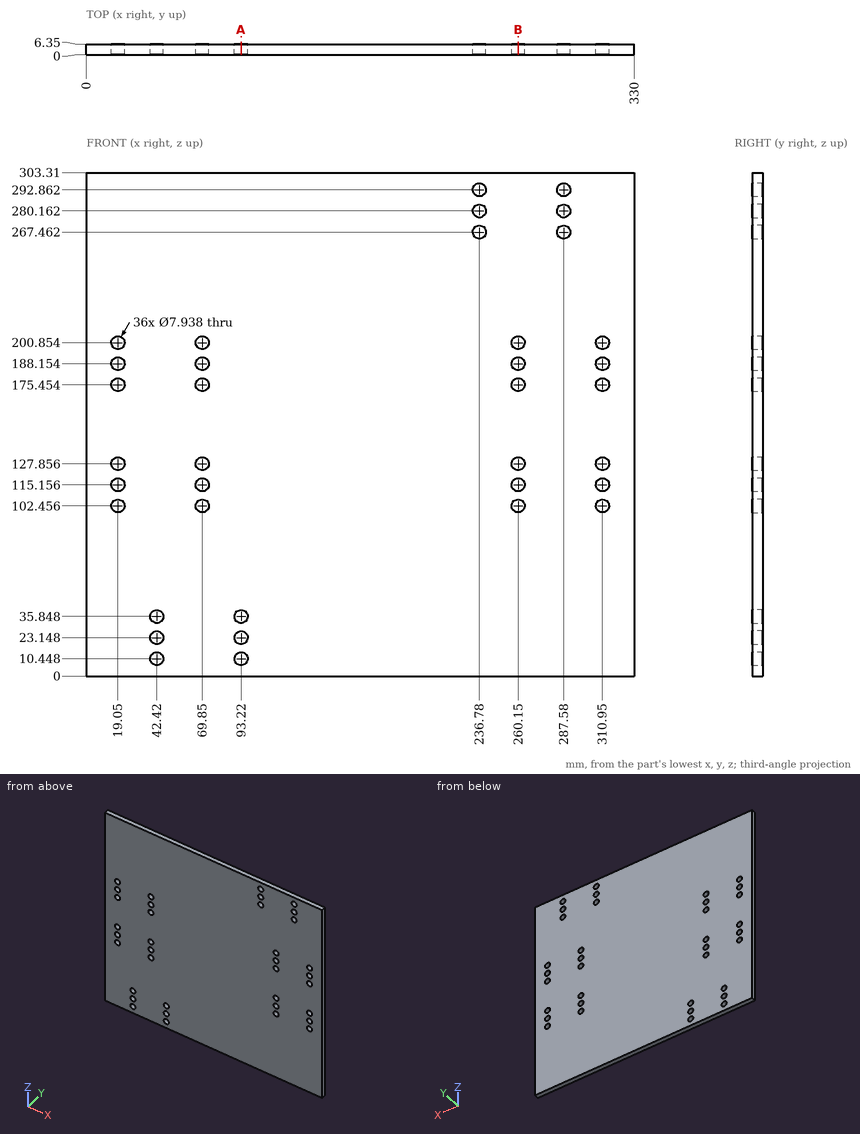
Geometry check sheet. Reference: drawing and pictorial views, mm from the part's lowest x, y, z. Give positions to 0.01 mm unless a question says otherwise; leave off trailing zeros. Loops run counter-clockwise (first coordinate to the right, second up) from the corner with the lowest first, then second, coordinate; pieces in that order, holes last. Notation, with made-up numbers: (-14, 71.5) -> (40, 71.5) arc R23 ccw to (40, 91.5) -> close; hole circle Ø6 at (88, 60). An arc over 180 degrees is marked (long way). Answer in a Markdown table with one row per item. Add a question column.
1) Cross-section at B-B on x = 260.15. State how many separate pieces and enclosed holes the cut face has, and give its area (3 significant figures).
2) Gauge pin test, flat end, axial feed: P1, Ø7, axis at x = 69.85, z = 188.154, coming from the +Y side. Record the tip position at first contact, or that the pin passes through.
3) Material ranges on probe 1 along X at (y, z) = (3.5, 281); probe 2 along X at (y, z) = (2.5, 280) (1 decimal); probe 3 along Z at (x, y) = (96, 2.75) (1 decimal), recorded low to high. Write a range as from..to.
4) Cross-section at A-A on x = 93.22. Record the boundary of the cut face in (y, z).
Outcome:
| question | item | result |
|---|---|---|
| 1 | separate pieces | 7 |
| 1 | enclosed holes | 0 |
| 1 | area | 1,620 mm^2 |
| 2 | P1 | passes through |
| 3 | probe 1 | x = 0..232.9, 240.66..283.7, 291.46..330 |
| 3 | probe 2 | x = 0..232.8, 240.7..283.6, 291.5..330 |
| 3 | probe 3 | z = 0..7.6, 13.3..20.3, 26..33, 38.7..303.3 |
| 4 | outline | (0, 0) -> (6.35, 0) -> (6.35, 6.48) -> (0, 6.48) -> close; (0, 14.42) -> (6.35, 14.42) -> (6.35, 19.18) -> (0, 19.18) -> close; (0, 27.12) -> (6.35, 27.12) -> (6.35, 31.88) -> (0, 31.88) -> close; (0, 39.82) -> (6.35, 39.82) -> (6.35, 303.31) -> (0, 303.31) -> close |
